Part model, mm, in its own coordinate system. Face numbers are marked on the shaded views. Coordinates: 2 decimals unless noted, no trailing zeros. Write each loop counter-clockwise with the first axis right and the second up, starting at its lowest first coordinate (ties: lowest second). Pieces come first, ordered by that corner, then holes. Notation, with made-up numbers: (74, -11.75) -> (133, -11.75) arc R16 cw to (133, 6.25) -> close; hole circle Ø7 at (62, 68). An arc over 180 degrees is marked (long way). Write item = value, one per line. Start each with the question number.
Q1. Band-saw the part on A-A, the plane y = -38. List the corners of the cut face in (x, z).
Q2. Probe line 1 (Y direction, x = -3, z = 1.8); line 2 (Y direction, x = 18, z = 2.4); line 3 (Y direction, x = 16.5, z = 0.95). List the from-to ranges inside material, lowest first.
Q3. Pull direction Y, two halves, no side cores. Call the marked faces 1, 2 and 3: released by +Y, released by -Y, zero draft, split by the parting line, or undercut.
Q4. Band-saw the part on B-B, the plane y = 0. List the corners of the cut face in (x, z), plus the area to 3 significant figures.
Q5. Pin check, flat tips, straight feed: P1, Ø11.5, axis at x = 0, y = 0, coming from the -Z side; P2, Ø6, axis at x = 2.5, y = 4, coming from the +Z side; P3, Ø2.5, axis at y = -20, z = 3.5, coming from the -X side. Stop position of each tip, or through.
Q6. Band-saw the part on C-C, the plane z = 2.6. List the corners of the cut face in (x, y), plus the area to 3 significant figures.
Q7. Band-saw the part on D-D, the plane y = -20. List the corners of the cut face in (x, z).
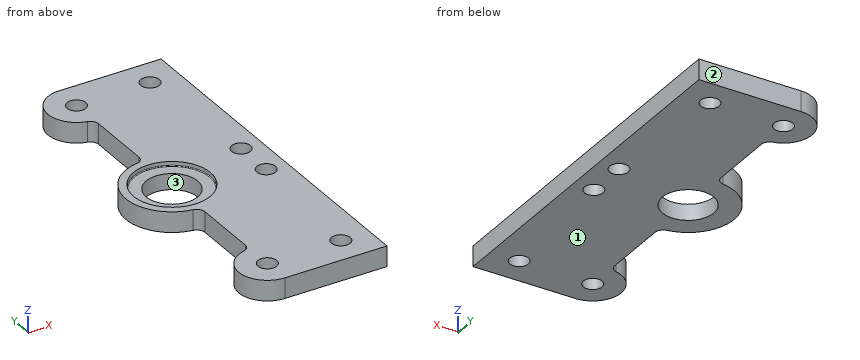
Autodesk Inventor part; units mm, degrees
ref_plane "YZ Plane" through (0, 0, 0) normal (1, 0, 0) x (0, 1, 0)
ref_plane "XZ Plane" through (0, 0, 0) normal (0, 1, 0) x (-1, 0, 0)
ref_plane "XY Plane" through (0, 0, 0) normal (0, 0, 1) x (1, 0, 0)
sketch "Sketch1" plane through (0, 0, 0) normal (0, 0, 1) x (1, 0, 0)
  circle A0 centre (0, 0) radius 20
  line L0 (-25, -45) -> (25, -45)
  line L1 (25, -45) -> (25, 45)
  line L2 (25, 45) -> (-25, 45)
  line L3 (-25, 45) -> (-25, -45)
  point P0 (-20, 0)
  point P1 (20, 0)
  dimension "d0" = 40
  dimension "d17" = 90
  dimension "d18" = 50
  dimension "d19" = 25
  dimension "d20" = 45
extrude "Extrusion1" add sketch "Sketch1" along normal blind 5 contours A0 | L3 L2 L1 L0
sketch "Sketch2" plane through (0, 0, 5) normal (0, 0, 1) x (1, 0, 0)
  line L0 (-25, 45) -> (-25, -45)
  line L1 (25, 45) -> (-25, 45)
  circle A0 centre (0, 0) radius 6.3
  dimension "d37" = 12.6
extrude "Extrusion2" cut sketch "Sketch2" against normal blind 5 from surface at 0
sketch "Sketch3" plane through (0, 0, 5) normal (0, 0, 1) x (1, 0, 0)
  circle A0 centre (0, 0) radius 4.5
  circle A1 centre (0, 0) radius 9.4
  dimension "d6" = 18.8
extrude "Extrusion3" cut sketch "Sketch3" against normal blind 1.1
fillet "Fillet1" radius 0.2 1 edges at (-9.4, 0, 3.9)
sketch "Sketch4" plane through (0, 0, 0) normal (0, 0, -1) x (-1, 0, 0)
  circle A0 centre (18, 38) radius 2.3
  circle A1 centre (-18, 38) radius 2.3
  circle A2 centre (18, -38) radius 2.3
  circle A3 centre (-18, -38) radius 2.3
  line L0 (-25, 45) -> (25, 45)
  line L1 (25, -45) -> (-25, -45)
  line L2 (25, 45) -> (25, -45)
  line L3 (-25, -45) -> (-25, 45)
  circle A4 centre (-20, 5) radius 2.3
  circle A5 centre (-20, -5) radius 2.3
  line L4 (-20, 5) -> (-20, -5)
  circle A6 centre (0, 0) radius 6.3
  circle A7 centre (0, 0) radius 11.3
  line L5 (0, 45) -> (0, 11.3) construction
  line L6 (0, -11.3) -> (0, -45) construction
  circle A8 centre (0, 38) radius 2.3
  circle A9 centre (0, -38) radius 2.3
  arc A10 (0, 31) -> (0, 45) centre (0, 38) ccw
  arc A11 (0, -45) -> (0, -31) centre (0, -38) ccw
  line L7 (0, 31) -> (0, 11.3)
  line L8 (0, -11.3) -> (0, -31)
  point P0 (-20, 0)
  dimension "d10" = 4.6
  dimension "d21" = 7
  dimension "d22" = 7
  dimension "d23" = 7
  dimension "d24" = 7
  dimension "d25" = 7
  dimension "d26" = 7
  dimension "d27" = 7
  dimension "d28" = 7
  dimension "d32" = 10
  dimension "d34" = 5
  dimension "d35" = 5
  dimension "d38" = 90
  dimension "d39" = 5
  dimension "d40" = 4.6
  dimension "d41" = 4.6
extrude "Extrusion4" cut sketch "Sketch4" against normal through all contours A0 | A1 | A2 | A3 | L0 L2 L1 A11 L8 A7 L7 A10 | A4 | A5 | A8 | A9
fillet "Fillet3" radius 2 4 edges at (0, 31, 2.5) (0, 11.3, 2.5) (0, -11.3, 2.5) (0, -31, 2.5)
equation "\"d22\" = d21"
equation "\"d23\" = d21"
equation "\"d24\" = d23"
equation "\"d26\" = d22"
equation "\"d27\" = d24"
equation "\"d28\" = d24"
equation "\"d40\" = d10"
equation "\"d41\" = d10"
properties part number "2113_Nut Stop Plate_V1" material "ABS Plastic"
Ans:
q1.outline = (-7, 0) -> (-2.3, 0) -> (-2.3, 5) -> (-7, 5) -> close; (2.3, 0) -> (15.7, 0) -> (15.7, 5) -> (2.3, 5) -> close; (20.3, 0) -> (25, 0) -> (25, 5) -> (20.3, 5) -> close
q2.line_1 = -44.32 to -31.68, -10.89 to -5.54, 5.54 to 10.89, 31.68 to 44.32
q2.line_2 = -45 to -40.3, -35.7 to -6.14, -3.86 to 3.86, 6.14 to 35.7, 40.3 to 45
q2.line_3 = -45 to -39.74, -36.26 to 36.26, 39.74 to 45
q3.face_1 = zero draft
q3.face_2 = released by +Y
q3.face_3 = undercut
q4.outline = (-11.3, 0) -> (-6.3, 0) -> (-6.3, 3.9) -> (-9.2, 3.9) arc R0.2 cw to (-9.4, 4.1) -> (-9.4, 5) -> (-11.3, 5) -> close; (6.3, 0) -> (25, 0) -> (25, 5) -> (9.4, 5) -> (9.4, 4.1) arc R0.2 cw to (9.2, 3.9) -> (6.3, 3.9) -> close
q4.area = 112 mm2
q5.P1 = through
q5.P2 = 3.9
q5.P3 = 0
q6.outline = (-1.7, -11.17) arc R2 cw to (0, -13.15) -> (0, -29.23) arc R2 cw to (-1.56, -31.18) arc R7 ccw to (0, -45) -> (25, -45) -> (25, 45) -> (0, 45) arc R7 ccw to (-1.56, 31.18) arc R2 cw to (0, 29.23) -> (0, 13.15) arc R2 cw to (-1.7, 11.17) arc R11.3 ccw to start; hole circle Ø12.6 at (0, 0); hole circle Ø4.6 at (0, -38); hole circle Ø4.6 at (0, 38); hole circle Ø4.6 at (18, -38); hole circle Ø4.6 at (18, 38); hole circle Ø4.6 at (20, -5); hole circle Ø4.6 at (20, 5)
q6.area = 2,380 mm2
q7.outline = (0, 0) -> (25, 0) -> (25, 5) -> (0, 5) -> close
